The figure shows three views and two pictorial views of one solid part (mm, origin at its lowest corner). Answer the questions. Give positions to 0.01 mm unless a question says otherwise; leave off trailing zeros. Write each loop counter-clockwise with the first axis right and the second up, starting at its lowest first coordinate (ties: lowest second). Pieces come first, ordered by that corner, then holes. Notation, with made-up numbers: (-35.5, 71.5) -> (2.5, 71.5) arc R33 cw to (2.5, 101.5) -> close; hole circle Ø8 at (49.5, -21.5). An arc over 180 degrees is marked (long way). Use a Markdown table: item, result.
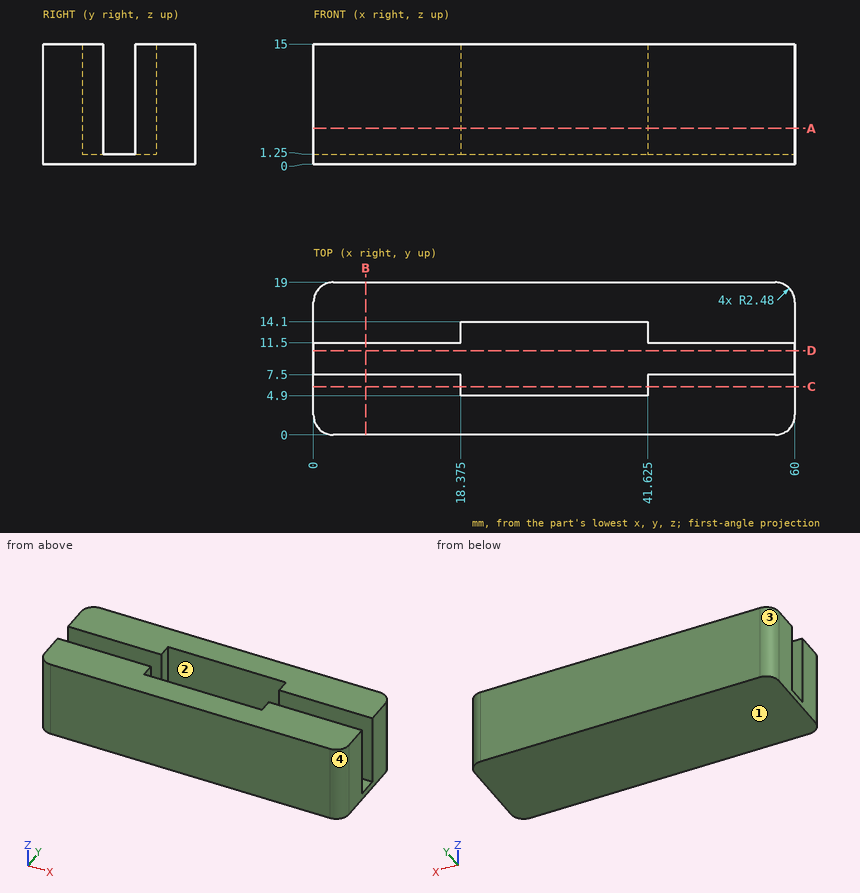
Item 1: For a pull along X with two mould halves and no side action, classify the marked faces 1, 2, 3 and 4 as +X half, -X half, draft (parallel to the pull), parting line (faces both ways), or undercut.
Return value:
| item | result |
|---|---|
| face 1 | draft |
| face 2 | undercut |
| face 3 | -X half |
| face 4 | +X half |
Item 2: A cutting plane is placed at D-D (y = 10.5). Give the vertices of the cut face in (x, z).
Return value:
| item | result |
|---|---|
| outline | (0, 0) -> (60, 0) -> (60, 1.25) -> (0, 1.25) -> close |
Item 3: A cutting plane is placed at A-A (z = 4.5). Give the vertices of the cut face in (x, y) (3 decimals), then the cut area to 3 significant figures.
Return value:
| item | result |
|---|---|
| outline | (0, 2.48) arc R2.48 ccw to (2.48, 0) -> (57.52, 0) arc R2.48 ccw to (60, 2.48) -> (60, 7.5) -> (41.625, 7.5) -> (41.625, 4.9) -> (18.375, 4.9) -> (18.375, 7.5) -> (0, 7.5) -> close; (0, 11.5) -> (18.375, 11.5) -> (18.375, 14.1) -> (41.625, 14.1) -> (41.625, 11.5) -> (60, 11.5) -> (60, 16.52) arc R2.48 ccw to (57.52, 19) -> (2.48, 19) arc R2.48 ccw to (0, 16.52) -> close |
| area | 774 mm^2 |
Item 4: Straight lines are drawn through the part: line 1 along Y through (x, z) = (5.5, 6.5); line 2 along Y through (x, z) = (23.5, 10.75); line 3 along X through (y, z) = (5.5, 5) (3 decimals). For each, find the intervals that lie inside material, in ascending order. Write a range as [from, to].
Return value:
| item | result |
|---|---|
| line 1 | [0, 7.5], [11.5, 19] |
| line 2 | [0, 4.9], [14.1, 19] |
| line 3 | [0, 18.375], [41.625, 60] |
Item 5: This flat-tipped pin is pushed along its axis until it touches: P1, Ø7.5, axis at x = 20, y = 8.5, coming from the +Z side. Where does it stop, or does it pass through?
Return value:
| item | result |
|---|---|
| P1 | z = 15 |
Item 6: A cutting plane is placed at C-C (y = 6). Give the vertices of the cut face in (x, z) (3 decimals).
Return value:
| item | result |
|---|---|
| outline | (0, 0) -> (60, 0) -> (60, 15) -> (41.625, 15) -> (41.625, 1.25) -> (18.375, 1.25) -> (18.375, 15) -> (0, 15) -> close |
Item 7: A cutting plane is placed at B-B (x = 6.5). Give the vertices of the cut face in (y, z), then the cut area to 3 significant figures.
Return value:
| item | result |
|---|---|
| outline | (0, 0) -> (19, 0) -> (19, 15) -> (11.5, 15) -> (11.5, 1.25) -> (7.5, 1.25) -> (7.5, 15) -> (0, 15) -> close |
| area | 230 mm^2 |
